For this review, take the finished solid that the model builds, in its own axes (mm). A direction names the side the tool comes from. Round coordinates to 2 decimals unless told otherwise and drop trailing zeros. Write each loop counter-clockwise with the first axis right and the second up, starting at its lowest first coordinate (ties: lowest second). Pieces come first, ordered by that corner, then holes.
from build123d import *

# Parameters (mm, degrees)
SKETCH1_R           = 16
BOSS_EXTRUDE1_DEPTH = 5
SKETCH3_R           = 15
CUT_EXTRUDE1_DEPTH  = 4
FILLET1_R           = 0.5
SKETCH7_W           = 5.268501054
SKETCH7_H           = 14.735182388
CUT_EXTRUDE2_DEPTH  = 11
SKETCH8_R           = 7.4
BOSS_EXTRUDE2_DEPTH = 3
SKETCH9_R           = 3.7
CUT_EXTRUDE3_DEPTH  = 3
SKETCH5_R           = 1.275
SKETCH6_R           = 1.3
FILLET3_R           = 0.4


with BuildPart() as part:
    # Sketch1 → Boss-Extrude1 (new body)
    with BuildSketch(Plane.XY):
        Circle(SKETCH1_R)
    extrude(amount=BOSS_EXTRUDE1_DEPTH)

    # Sketch3 → Cut-Extrude1 (cut)
    with BuildSketch(Plane.XY.offset(5)):
        Circle(SKETCH3_R)
    extrude(amount=-CUT_EXTRUDE1_DEPTH, mode=Mode.SUBTRACT)

    # Fillet1
    fillet1_edges = [part.edges().sort_by_distance(p)[0] for p in [
        (-15, 0, 1),
    ]]
    fillet(fillet1_edges, radius=FILLET1_R)

    # Sketch7 → Cut-Extrude2 (cut)
    with BuildSketch(Plane.XY.offset(13)):
        with Locations((-14.456252894, -1.028256592)):
            Rectangle(SKETCH7_W, SKETCH7_H)
    cut_extrude2 = extrude(amount=-CUT_EXTRUDE2_DEPTH, mode=Mode.SUBTRACT)

    # Mirror1: Cut-Extrude2 across plane
    add(cut_extrude2.mirror(Plane(origin=(0, 0, 0), x_dir=(0, 0, 1), z_dir=(1, 0, 0))), mode=Mode.SUBTRACT)

    # Sketch8 → Boss-Extrude2 (add)
    with BuildSketch(Plane.XY.offset(1)):
        Circle(SKETCH8_R)
    extrude(amount=BOSS_EXTRUDE2_DEPTH)

    # Sketch9 → Cut-Extrude3 (cut)
    with BuildSketch(Plane.XY.offset(4)):
        Circle(SKETCH9_R)
    extrude(amount=-CUT_EXTRUDE3_DEPTH, mode=Mode.SUBTRACT)

    # Sketch5 → Loft1 section 0
    with BuildSketch(Plane.XY.offset(1)):
        Circle(SKETCH5_R)
    # Sketch6 → Loft1 section 1
    with BuildSketch(Plane.XY.offset(13)):
        Circle(SKETCH6_R)
    loft()

    # Fillet3
    fillet3_edges = [part.edges().sort_by_distance(p)[0] for p in [
        (-1.275, 0, 1),
    ]]
    fillet(fillet3_edges, radius=FILLET3_R)


solid = part.part
(1) For pin 1 Ø1.1 at (x, y) = (-13.5, -3.5) entering from +Z; pin 2 Ø6 at (x, z) = (7, 6.5) entering from -Y; pin 3 Ø8.5 at (x, y) = (4, -10.5) entering from +Z, all flat-tipped, find the tip position at first contact; note any pin that passes through.
Geometry check:
pin 1: stops at z = 1
pin 2: stops at y = -15.38
pin 3: stops at z = 5
(2) We need section B-B, the plane z = 9.25. Give the boundary of the cut face in (x, y).
Geometry check:
outline: circle Ø2.58 at (0, 0)
(3) We need section A-A, the plane z = 6.75. Give the boundary of the cut face in (x, y).
Geometry check:
outline: circle Ø2.57 at (0, 0)
(4) For faces 1 (the face through (0, 0, 0)), 2 (the face through (1, -2, 1)), 3 (the face through (-13, -8.396, 4)), list the 3-axis set-ups (+Z, -Z, +X, -X, +Y, -Y) from which the entire face can be reached by the end or side of a thin tool; tool diameter is ignored.
Geometry check:
face 1: -Z, +X, -X, +Y, -Y
face 2: +Z
face 3: +Z, +X, -X
(5) Mouldability with a two-part tool opening along Y and no side actions: class faces 4 (the face through (-15.985, 0.703, 1.354)), 5 (the face through (3, -3, 4)), 6 (the face through (-1.16, 15.13, 5)) as pulls with the +Y half, pulls with the -Y half, needs draft (parallel to the pull), parting line crosses it, or undercut.
Geometry check:
face 4: parting line crosses it
face 5: undercut
face 6: needs draft
(6) For line 1 along Y through (x, z) = (0, 3.75); line 2 along Z through (x, y) = (-2, 2); line 3 along Y through (x, z) = (10, 3), list the stretches that pass through material, from the lowest coordinate up.
Geometry check:
line 1: y = -16 to -15, -7.4 to -3.7, -1.28 to 1.28, 3.7 to 7.4, 15 to 16
line 2: z = 0 to 1
line 3: y = -12.49 to -11.18, 11.18 to 12.49
